Here's how the part is built. I have some questions about the finished solid (model axes, mm). A direction names the side the tool comes from. Round coordinates to 2 decimals unless told otherwise and drop trailing zeros. Order: outer loops, then holes, each group sorted by start corner. A loop starts at its lowest first (then second) coordinate and runs counter-clockwise, first axis right, second up. Notation, with made-up numbers: (5.25, 72.25) -> (38.25, 72.25) arc R6 cw to (38.25, 77.25) -> close; hole circle Ø7 at (-18.75, -40). An arc over 180 degrees is marked (long way). Use a Markdown table: item, result. Add a question column.
from build123d import *

# Parameters (mm, degrees)
BOSS_EXTRUDE1_DEPTH = 30
SKETCH2_R           = 4
BOSS_EXTRUDE2_DEPTH = 5
CUT_EXTRUDE1_DEPTH  = 27
SKETCH4_R           = 1.25
CUT_EXTRUDE2_DEPTH  = 10


with BuildPart() as part:
    # Sketch1 → Boss-Extrude1 (new body)
    with BuildSketch(Plane(origin=(0, 0, 0), x_dir=(1, 0, 0), z_dir=(0, 1, 0))):
        with BuildLine():
            Line((-25, 15), (-25, 0))
            Line((-25, 0), (25, 0))
            Line((25, 0), (25, 15))
            ThreePointArc((25, 15), (0, 19.616515847), (-25, 15))
        make_face()
    extrude(amount=BOSS_EXTRUDE1_DEPTH)

    # Sketch2 → Boss-Extrude2 (add)
    with BuildSketch(Plane(origin=(0, 30, 0), x_dir=(1, 0, 0), z_dir=(0, 1, 0))):
        with Locations(Location((-10, 10, 0), (0, 0, 270))):
            Circle(SKETCH2_R)
        with Locations(Location((10, 10, 0), (0, 0, 270))):
            Circle(SKETCH2_R)
    extrude(amount=BOSS_EXTRUDE2_DEPTH)

    # Sketch3 → Cut-Extrude1 (cut)
    with BuildSketch(Plane.XZ.offset(-30)):
        Polygon((0, -7), (-3.031088913, -8.75), (-3.031088913, -12.25), (0, -14), (3.031088913, -12.25), (3.031088913, -8.75), align=None)
    extrude(amount=CUT_EXTRUDE1_DEPTH, mode=Mode.SUBTRACT)

    # Sketch4 → Cut-Extrude2 (cut)
    with BuildSketch(Plane.XZ):
        with Locations(Location((0, -10.5, 0), (0, 0, 270))):
            Circle(SKETCH4_R)
    extrude(amount=-CUT_EXTRUDE2_DEPTH, mode=Mode.SUBTRACT)


solid = part.part
(1) I want a section at D-D on z = -5.25. List the corners of the cut face in (x, y) for me.
(2) Please list where these lines run through material, in increasing order: probe 1 along X at (y, z) = (1.75, -10.5); probe 2 along Y at (x, z) = (20, -15); probe 3 along Z at (x, y) = (-2.5, 10). Write a range as from..to.
(3) If we mould it in two halves opening along Z, with no side actions, what happens to faces 1 (the flat face through (3.031, 17, -11)), 2 (the cylindrical face through (-12.4, 32.5, -13.2)), 3 (the flat face through (-1.49, 16.69, -7.86)), 4 (the flat face through (-10, 35, -10))? For each: pulls with the +Z half, pulls with the -Z half, needs draft (parallel to the pull), parting line crosses it, or undercut.
(4) I want a section at A-A on z = -10. List the corners of the cut face in (x, y) for me.
(5) I want a section at C-C on x = -12.5. List the corners of the cut face in (y, z) for me.
(6) On a 3-axis mill with a long thin cutter (end or side, diameter ignored), from which of +Z, -Z, +X, -X, +Y, -Y can I reach the whole of each face in a straight line? I mean faces 5 (the flat face through (1.54, 16.69, -7.89)), 6 (the cylindrical face through (0.358, 14.79, -19.616)). Say none if no direction works.
(7) I want a section at B-B on y = 20. List the corners of the cut face in (x, z) for me, and give its area (3 significant figures).
(8) I'm going to push flat-ended pins straight in: P1, Ø3, axis at x = 0, z = -10.5, coming from the +Y side; P2, Ø2, axis at x = 14.5, y = 24, coming from the -Z side; P3, Ø5, axis at x = -1, z = -10, coming from the +Y side. Where does each tip first touch, or does it pass through?
Output:
| question | item | result |
|---|---|---|
| 1 | outline | (-25, 0) -> (25, 0) -> (25, 30) -> (-25, 30) -> close |
| 2 | probe 1 | -25..-1.25, 1.25..25 |
| 2 | probe 2 | 0..30 |
| 2 | probe 3 | -19.57..-12.56, -8.44..0 |
| 3 | face 1 | undercut |
| 3 | face 2 | parting line crosses it |
| 3 | face 3 | undercut |
| 3 | face 4 | needs draft |
| 4 | outline | (-25, 0) -> (-1.15, 0) -> (-1.15, 3) -> (-3.03, 3) -> (-3.03, 30) -> (-6, 30) -> (-6, 35) -> (-14, 35) -> (-14, 30) -> (-25, 30) -> close; (1.15, 0) -> (25, 0) -> (25, 30) -> (14, 30) -> (14, 35) -> (6, 35) -> (6, 30) -> (3.03, 30) -> (3.03, 3) -> (1.15, 3) -> close |
| 5 | outline | (0, -18.49) -> (30, -18.49) -> (30, -13.12) -> (35, -13.12) -> (35, -6.88) -> (30, -6.88) -> (30, 0) -> (0, 0) -> close |
| 6 | face 5 | +Y |
| 6 | face 6 | -Z, +Y, -Y |
| 7 | outline | (-25, -15) arc R70 ccw to (25, -15) -> (25, 0) -> (-25, 0) -> close; hole (-3.03, -12.25) -> (0, -14) -> (3.03, -12.25) -> (3.03, -8.75) -> (0, -7) -> (-3.03, -8.75) -> close |
| 7 | area | 873 mm² |
| 8 | P1 | y = 3 |
| 8 | P2 | z = -18.3 |
| 8 | P3 | y = 30 |
